The listing builds one solid part. Answer for the finished solid, in the listing's coordinates (mm). A direction names the side the tool comes from. Round coordinates to 2 decimals unless told otherwise and drop trailing zeros. Write each loop counter-clockwise with the first axis right and the second up, starting at its lowest first coordinate (ties: lowest second). Pieces come first, ordered by that corner, then holes. Notation, with made-up numbers: (17.25, -33) - (32.25, -33) arc R8 cw to (32.25, -19) - close; hole circle Ø3 at (71.5, 4.5). An arc over 180 degrees is marked (long way). Answer as CSV lines item,"result". Start each with the question number.
Item 1: A cutting plane is placed at D-D on x = 71. Determine the outline of the cut face in (y, z), and give its area (3 significant figures).
Item 2: A cutting plane is placed at C-C on z = 3. Determine the outline of the cut face in (x, y).
Item 3: Flat-ended cylindrical pins translate along their axes: pin 1 (1.8 mm diameter, centred on x = 0.55, z = -8.22, fed in from -Y); pin 2 (3.5 mm diameter, centred on y = -23, z = 8.78, fed in from +X); pin 3 (2.5 mm diameter, centred on x = -7.45, z = -8.22, fed in from +Y); pin 4 (8 mm diameter, centred on y = -12, z = 7, fed in from -X). Find the tip coordinate at first contact, or state that the pin passes through.
Item 4: Which of the six approach directions +Z, -Z, +X, -X, +Y, -Y give full straight-line access (tool end or side, diameter ignored) to faces 1 (the flat face through (78, -35, 2)), 2 (the flat face through (10.051, 10, 2))?
Item 5: A cutting plane is placed at B-B on y = -8.5. Determine the outline of the cut face in (x, z).
Item 6: Straight lines are drawn through the part: line 1 along X through (y, z) = (-4, 0); line 2 along X through (y, z) = (-7.5, 5.5); line 3 along X through (y, z) = (-21.5, -2). For each, find the intervals that lie inside material, in ascending order. Write a range as [from, to].
Item 7: A cutting plane is placed at A-A on y = -23. Determine the outline of the cut face in (x, z).
Item 8: For a pull along Z with two mould halves and no side action, classify faces 3 (the cylindrical face through (46.052, 11.037, -5.286)), 4 (the flat face through (46, 8, -13.22)), 5 (the cylindrical face through (9.475, 2.878, 8.163)), 6 (the flat face through (18.051, -10, 2)) as pulls with the +Z half, pulls with the -Z half, needs draft (parallel to the pull), parting line crosses it, or undercut.
Autodesk Inventor part; units mm, degrees
ref_plane "YZ Plane" through (0, 0, 0) normal (1, 0, 0) x (0, 1, 0)
ref_plane "XZ Plane" through (0, 0, 0) normal (0, 1, 0) x (-1, 0, 0)
ref_plane "XY Plane" through (0, 0, 0) normal (0, 0, 1) x (1, 0, 0)
sketch "Esquisse1" plane through (0, 0, 0) normal (0, 1, 0) x (-1, 0, 0)
  line L0 (11.9492, 16.7797) -> (-18.0508, 16.7797)
  line L1 (-18.0508, 16.7797) -> (-18.0508, -13.2203)
  line L2 (-18.0508, -13.2203) -> (11.9492, -13.2203)
  line L3 (11.9492, -13.2203) -> (11.9492, 16.7797)
  point P0 (0, 0)
  dimension "d0" = 30
  dimension "d1" = 30
extrude "Extrusion1" add sketch "Esquisse1" along normal blind 5
sketch "Esquisse2" plane through (0, 5, 0) normal (0, 1, 0) x (1, 0, 0)
  line L0 (-11.9492, 17.2203) -> (-2.9492, 17.2203)
  line L1 (-11.9492, -16.7797) -> (-11.9492, 17.2203)
  line L2 (-11.9492, -16.7797) -> (-2.9492, -16.7797)
  line L3 (-2.9492, -15.7797) -> (-2.9492, -16.7797)
  line L4 (-2.9492, -15.7797) -> (5.0508, -15.7797)
  line L5 (5.0508, -15.7797) -> (5.0508, -16.7797)
  line L6 (5.0508, -16.7797) -> (13.0508, -16.7797)
  line L7 (13.0508, 17.2203) -> (13.0508, -16.7797)
  line L8 (5.0508, 17.2203) -> (13.0508, 17.2203)
  line L9 (5.0508, 16.2203) -> (5.0508, 17.2203)
  line L10 (-2.9492, 16.2203) -> (5.0508, 16.2203)
  line L11 (-2.9492, 16.2203) -> (-2.9492, 17.2203)
  circle A0 centre (-7.4492, 0.2203) radius 1
  circle A1 centre (-7.4492, 8.2203) radius 1
  circle A2 centre (-7.4492, -7.7797) radius 1
  circle A3 centre (0.5508, -7.7797) radius 1
  circle A4 centre (8.5508, 0.2203) radius 1
  circle A5 centre (8.5508, 8.2203) radius 1
  circle A6 centre (8.5508, -7.7797) radius 1
  circle A7 centre (0.5508, 8.2203) radius 1
  arc A8 (3.5508, -2.4254) -> (3.5508, 2.8661) centre (0.5508, 0.2203) ccw
  line L12 (3.5508, -2.4254) -> (3.5508, -4.7797)
  line L13 (3.5508, -4.7797) -> (-2.4492, -4.7797)
  line L14 (-2.4492, -4.7797) -> (-2.4492, -2.4254)
  arc A9 (-2.4492, 2.8661) -> (-2.4492, -2.4254) centre (0.5508, 0.2203) ccw
  line L15 (-2.4492, 2.8661) -> (-2.4492, 5.2203)
  line L16 (-2.4492, 5.2203) -> (3.5508, 5.2203)
  line L17 (3.5508, 5.2203) -> (3.5508, 2.8661)
  circle A10 centre (8.5508, 8.2203) radius 1
  circle A11 centre (8.5508, 0.2203) radius 1
  circle A12 centre (8.5508, -7.7797) radius 1
  circle A13 centre (0.5508, -7.7797) radius 1
  circle A14 centre (-7.4492, -7.7797) radius 1
  circle A15 centre (-7.4492, 0.2203) radius 1
  circle A16 centre (-7.4492, 8.2203) radius 1
  circle A17 centre (0.5508, 8.2203) radius 1
  point P0 (0, 0)
extrude "Extrusion2" cut sketch "Esquisse2" against normal through all contours A0 | A1 | A2 | A3 | A4 | A5 | A6 | A7
sketch "Esquisse3" plane through (0, 5, 0) normal (0, 1, 0) x (1, 0, 0)
  line L0 (18.0508, 13.2203) -> (-11.9492, 13.2203)
  line L1 (10.0508, -16.7797) -> (10.0508, 13.2203)
  line L2 (-11.9492, -16.7797) -> (18.0508, -16.7797)
  line L3 (18.0508, -16.7797) -> (18.0508, 13.2203)
  line L4 (10.0508, 13.2203) -> (18.0508, 13.2203)
  line L5 (18.0508, 13.2203) -> (18.0508, -16.7797)
  line L6 (18.0508, -16.7797) -> (10.0508, -16.7797)
  line L7 (10.0508, -16.7797) -> (10.0508, 13.2203)
  point P0 (0, 0)
  dimension "d7" = 8
extrude "Extrusion3" add sketch "Esquisse3" along normal blind 10
fillet "Congé4" radius 2 1 edges at (10.0508, 5, 1.7797)
sketch "Esquisse5" plane through (-11.9492, 0, 16.7797) normal (0, 0, 1) x (1, 0, 0)
  circle A0 centre (59.5, -23) radius 30
  line L0 (30, 0) -> (30, 15)
  line L1 (30, 15) -> (95, 15)
  line L2 (95, 15) -> (95, -35)
  line L3 (30, -17.5456) -> (30, 15)
  arc A1 (86.9955, -35) -> (30, -17.5456) centre (59.5, -23) ccw
  line L4 (95, -35) -> (86.9955, -35)
  line L5 (32.0045, -35) -> (30, -35)
  point P0 (11.9492, 0)
  dimension "d17" = 65
  dimension "d18" = 50
extrude "Extrusion4" add sketch "Esquisse5" against normal blind 30 contours A0 L3 L0 L1 L2 L4
fillet "Congé5" radius 2 1 edges at (18.0508, 0, 1.7797)
fillet "Congé6" radius 2 1 edges at (10.0508, 15, 1.7797)
fillet "Congé7" radius 2 1 edges at (83.0508, 15, 1.7797)
fillet "Congé8" radius 2 1 edges at (83.0508, -35, 1.7797)
sketch "Esquisse6" plane through (83.0508, 13, 16.7797) normal (1, 0, 0) x (0, 0, -1)
  circle A0 centre (8, -36) radius 1.5
  circle A1 centre (22, -36) radius 1.5
  line L0 (0, -46) -> (0, 0)
  line L1 (30, 0) -> (30, -46)
  line L2 (171, -6) -> (-4, -6)
  line L3 (171, -66) -> (-4, -66)
  point P0 (16.7797, -13)
  dimension "d25" = 3
  dimension "d26" = 3
  dimension "d27" = 8
  dimension "d28" = 8
  dimension "d29" = 30
  dimension "d30" = 30
extrude "Extrusion5" cut sketch "Esquisse6" against normal through all
sketch "Esquisse7" plane through (0, 15, 0) normal (0, 1, 0) x (1, 0, 0)
  circle A0 centre (47.5508, 5.2203) radius 1.5
  circle A1 centre (47.5508, -8.7797) radius 1.5
  line L0 (12.0508, -16.7797) -> (81.0508, -16.7797)
  line L1 (12.0508, 13.2203) -> (81.0508, 13.2203)
  line L2 (17.5508, 154.2203) -> (17.5508, -20.7797)
  point P0 (0, 0)
  dimension "d33" = 3
  dimension "d34" = 3
  dimension "d35" = 8
  dimension "d36" = 8
  dimension "d37" = 30
  dimension "d38" = 30
extrude "Extrusion6" cut sketch "Esquisse7" against normal through all
properties part number "support-trappe"
Geometry says:
1,outline,"(-4.29, -13.22) - (15, -13.22) - (15, 16.78) - (-4.29, 16.78) - close"
1,area,"579 mm^2"
2,outline,"(-11.95, 0) - (16.05, 0) arc R2 cw to (18.05, -2) - (18.05, -17.55) arc R30 cw (long way) to (75.05, -35) - (81.05, -35) arc R2 ccw to (83.05, -33) - (83.05, 13) arc R2 ccw to (81.05, 15) - (12.05, 15) arc R2 ccw to (10.05, 13) - (10.05, 7) arc R2 cw to (8.05, 5) - (-11.95, 5) - close"
3,pin 1,"passes through"
3,pin 2,"stops at x = 83.05"
3,pin 3,"stops at y = 5"
3,pin 4,"stops at x = 18.05"
4,face 1,"+Z, -Z, +X, -X, -Y"
4,face 2,"+Z, -Z, -X, +Y"
5,outline,"(18.05, -13.22) - (21.29, -13.22) - (21.29, 16.78) - (18.05, 16.78) - close; (73.81, -13.22) - (83.05, -13.22) - (83.05, 16.78) - (73.81, 16.78) - close"
6,line 1,"x = [18.05, 24.33], [70.77, 83.05]"
6,line 2,"x = [18.05, 21.87], [73.24, 83.05]"
6,line 3,"x = [77.51, 83.05]"
7,outline,"(77.55, -13.22) - (83.05, -13.22) - (83.05, -6.72) - (77.55, -6.72) - close; (77.55, -3.72) - (83.05, -3.72) - (83.05, 7.28) - (77.55, 7.28) - close; (77.55, 10.28) - (83.05, 10.28) - (83.05, 16.78) - (77.55, 16.78) - close"
8,face 3,"undercut"
8,face 4,"pulls with the -Z half"
8,face 5,"undercut"
8,face 6,"needs draft"
